from build123d import *

# Parameters (mm, degrees)
F1_DEPTH = 25.4
F2_R     = 5.08


with BuildPart() as f1:
    # F0 (on Top) → F1 (new body)
    with BuildSketch(Plane.XY):
        Polygon((14.8781485382, 63.5), (-48.6218514618, 63.5), (-48.6218514618, -31.75), (-80.3718514618, -31.75), (-80.3718514618, -127), (-32.7468514618, -127), (-32.7468514618, 0), (-0.9968514618, 0), (-0.9968514618, -127), (46.6281485382, -127), (46.6281485382, -31.75), (14.8781485382, -31.75), align=None)
    extrude(amount=F1_DEPTH)

    # F2
    f2_edges = [f1.edges().sort_by_distance(p)[0] for p in [
        (14.878149, 15.875, 25.4),
        (-48.621851, 15.875, 25.4),
        (-48.621851, 15.875, 0),
        (14.878149, 15.875, 0),
        (14.878149, -31.75, 12.7),
        (-48.621851, -31.75, 12.7),
        (-80.371851, -31.75, 12.7),
        (-80.371851, -79.375, 25.4),
        (-80.371851, -79.375, 0),
        (-56.559351, -127, 25.4),
        (-80.371851, -127, 12.7),
        (22.815649, -127, 25.4),
        (46.628149, -79.375, 25.4),
        (-0.996851, -127, 12.7),
        (46.628149, -127, 12.7),
        (22.815649, -127, 0),
        (-32.746851, -127, 12.7),
        (-16.871851, 0, 25.4),
        (-32.746851, -63.5, 25.4),
        (-0.996851, -63.5, 25.4),
        (46.628149, -31.75, 12.7),
        (-0.996851, -63.5, 0),
        (-16.871851, 0, 0),
        (46.628149, -79.375, 0),
        (-32.746851, -63.5, 0),
        (-0.996851, 0, 12.7),
        (-32.746851, 0, 12.7),
        (-56.559351, -127, 0),
        (-64.496851, -31.75, 0),
        (-64.496851, -31.75, 25.4),
        (30.753149, -31.75, 0),
        (30.753149, -31.75, 25.4),
    ]]
    fillet(f2_edges, radius=F2_R)


solid = f1.part
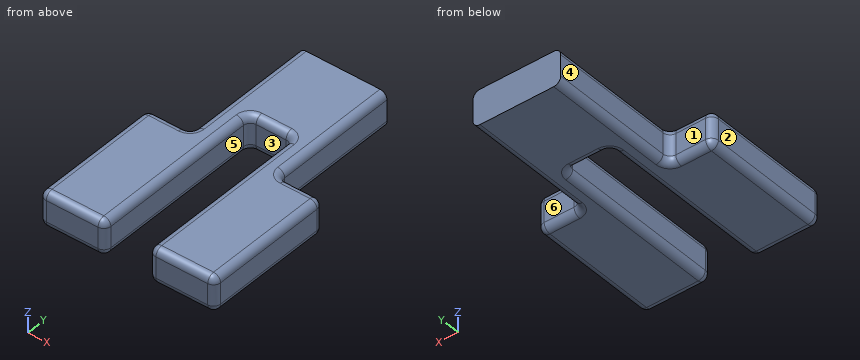
CAD build for the part. Positions are in the model's coordinates, mm. Face numbers are marked on the shaded views. A direction names the side the tool comes from. Round coordinates to 2 decimals unless told otherwise and drop trailing zeros. Order: outer loops, then holes, each group sorted by start corner. A loop starts at its lowest first (then second) coordinate and runs counter-clockwise, first axis right, second up. Notation, with made-up numbers: M 32,77.5 L 85,77.5 A35 cw 85,115.5 Z; hole C -25,50 d1. An arc over 180 degrees is marked long. Use one line per item in the form item = value.
Q1. Probe L1, parallel to X at y = -111.5, z = 17.25; L2, parallel to X at y = -12, z = 6; L3, parallel to Y at x = 35, z = 14.5. List the from-to ranges inside material, lowest first.
Recorded:
L1 = -80.37 to -32.75, -1 to 46.63
L2 = -48.62 to -32.75, -1 to 14.88
L3 = -127 to -31.75
Q2. Saw through at C-C on x = 23. Give the cut face in (y, z), then the cut area to 3 significant figures.
Recorded:
outline = M -127,5.08 A5.08 ccw -121.92,0 L -36.83,0 A5.08 ccw -31.75,5.08 L -31.75,20.32 A5.08 ccw -36.83,25.4 L -121.92,25.4 A5.08 ccw -127,20.32 Z
area = 2,400 mm^2
Q3. Which spindle directions (+Z, -Z, +X, -X, +Y, -Y) get a long thin tool onto all of the face, cutting with end or side? Do the marked faces 4, 5 and 6. Say none if no direction does.
Recorded:
face_4 = +Z, -Z, -X, +Y
face_5 = +Z, -Z, -Y
face_6 = +Z, -Z, +X, +Y
Q4. Two-plate mould, pull along X, no slides. Class the marked faces 1, 2 and 3: +X half, -X half, draft (parallel to the pull), parting line (faces both ways), or undercut.
Recorded:
face_1 = draft
face_2 = -X half
face_3 = undercut
Q5. Saw through at A-A on y = -42. Give the cut face in (x, z).
Recorded:
outline = M -80.37,5.08 A5.08 ccw -75.29,0 L -37.83,0 A5.08 ccw -32.75,5.08 L -32.75,20.32 A5.08 ccw -37.83,25.4 L -75.29,25.4 A5.08 ccw -80.37,20.32 Z; M -1,5.08 A5.08 ccw 4.08,0 L 41.55,0 A5.08 ccw 46.63,5.08 L 46.63,20.32 A5.08 ccw 41.55,25.4 L 4.08,25.4 A5.08 ccw -1,20.32 Z
Q6. Flat gauge pins, fed straight in: P1, Ø3, axis at y = 28, z = 23, coming from the +X side; P2, Ø3, axis at x = 3, z = 7, coming from the -Y side; P3, Ø5, axis at y = -19, z = 18.5, coming from the -X side; P4, Ø1, axis at x = 1, z = 5, coming from the -Y side. Where does each tip first touch, or does it go through?
Recorded:
P1 = 14.74
P2 = -127
P3 = -48.62
P4 = -126.29
Q7. Saw through at D-D on z = 15. Give the cut face in (x, y).
Recorded:
outline = M -80.37,-121.92 A5.08 ccw -75.29,-127 L -37.83,-127 A5.08 ccw -32.75,-121.92 L -32.75,-5.08 A5.08 cw -27.67,0 L -6.08,0 A5.08 cw -1,-5.08 L -1,-121.92 A5.08 ccw 4.08,-127 L 41.55,-127 A5.08 ccw 46.63,-121.92 L 46.63,-36.83 A5.08 ccw 41.55,-31.75 L 19.96,-31.75 A5.08 cw 14.88,-26.67 L 14.88,63.5 L -48.62,63.5 L -48.62,-26.67 A5.08 cw -53.7,-31.75 L -75.29,-31.75 A5.08 ccw -80.37,-36.83 Z
Q8. Saw through at B-B on y = 40. Give the cut face in (x, z), then the cut area to 3 significant figures.
Recorded:
outline = M -48.62,5.08 A5.08 ccw -43.54,0 L 9.8,0 A5.08 ccw 14.88,5.08 L 14.88,20.32 A5.08 ccw 9.8,25.4 L -43.54,25.4 A5.08 ccw -48.62,20.32 Z
area = 1,590 mm^2
